from build123d import *

# Parameters (mm, degrees)
SKETCH_1_R      = 2
EXTRUDE_1_DEPTH = 3
FILLET_1_R      = 2
FILLET_2_R      = 5


with BuildPart() as part:
    # ｽｹｯﾁ1 → ﾎﾞｽ - 押し出し1 (new body)
    with BuildSketch(Plane(origin=(0, 0, 0), x_dir=(1, 0, 0), z_dir=(0, 1, 0))):
        Polygon((0, 20), (0, 160), (-10, 160), (-13.241161391, 160), (-45.078057301, 128.16310409), (-128.16310409, 45.078057301), (-160, 13.241161391), (-160, 10), (-160, 0), (-20, 0), align=None)
        with Locations(Location((-5, 25, 0), (0, 0, 270))):
            Circle(SKETCH_1_R, mode=Mode.SUBTRACT)
        with Locations(Location((-5, 90, 0), (0, 0, 270))):
            Circle(SKETCH_1_R, mode=Mode.SUBTRACT)
        with Locations(Location((-90, 5, 0), (0, 0, 270))):
            Circle(SKETCH_1_R, mode=Mode.SUBTRACT)
        with Locations(Location((-25, 5, 0), (0, 0, 270))):
            Circle(SKETCH_1_R, mode=Mode.SUBTRACT)
        with Locations(Location((-68.942911166, 97.227182413, 0), (0, 0, 270))):
            Circle(SKETCH_1_R, mode=Mode.SUBTRACT)
        with Locations(Location((-30.0520382, 58.336309448, 0), (0, 0, 270))):
            Circle(SKETCH_1_R, mode=Mode.SUBTRACT)
        with Locations(Location((-58.336309448, 30.0520382, 0), (0, 0, 270))):
            Circle(SKETCH_1_R, mode=Mode.SUBTRACT)
        with Locations(Location((-97.227182413, 68.942911166, 0), (0, 0, 270))):
            Circle(SKETCH_1_R, mode=Mode.SUBTRACT)
        with Locations(Location((-5, 155, 0), (0, 0, 270))):
            Circle(SKETCH_1_R, mode=Mode.SUBTRACT)
        with Locations(Location((-155, 5, 0), (0, 0, 270))):
            Circle(SKETCH_1_R, mode=Mode.SUBTRACT)
        Polygon((-82.201163313, 13.258252147), (-13.258252147, 82.201163313), (-45.078057301, 114.020968466), (-114.020968466, 45.078057301), align=None, mode=Mode.SUBTRACT)
    extrude(amount=EXTRUDE_1_DEPTH)

    # ﾌｨﾚｯﾄ1
    fillet_1_edges = [part.edges().sort_by_distance(p)[0] for p in [
        (-13.241161391, 1.5, -160),
        (0, 1.5, -160),
        (0, 1.5, -20),
        (-20, 1.5, 0),
        (-160, 1.5, 0),
        (-160, 1.5, -13.241161391),
    ]]
    fillet(fillet_1_edges, radius=FILLET_1_R)

    # ﾌｨﾚｯﾄ2
    fillet_2_edges = [part.edges().sort_by_distance(p)[0] for p in [
        (-82.201163313, 1.5, -13.258252147),
        (-13.258252147, 1.5, -82.201163313),
        (-45.078057301, 1.5, -114.020968466),
        (-114.020968466, 1.5, -45.078057301),
    ]]
    fillet(fillet_2_edges, radius=FILLET_2_R)


solid = part.part
Read the model definition and answer for the solid it produces. Units are mm, in the model's axes. A direction names the side the tool comes from. Give positions to 0.01 mm unless a question says otherwise; leave off trailing zeros. Write each loop counter-clockwise with the first axis right and the second up, starting at its lowest first coordinate (ties: lowest second). Pieces come first, ordered by that corner, then holes. Notation, with made-up numbers: M -6.75,59 L 16.25,59 A19 cw 16.25,74 Z; hole C 49.25,86 d3. An arc over 180 degrees is marked long. One line per item, written item: value. Start each with the question number.
(1) Find section A-A (z = -5). Determine the outline of the cut face in (x, y).
(2) A tool of negligible diameter and unlimited length cuts with its end or side. For faces 5 (the flat face through (-46, 0, -46)), 6 (the flat face through (-28.995, 1.479, -97.938)), from which of +Z, -Z, +X, -X, +Y, -Y can it reach the whole face along a straight path? Write none if from no direction.
(3) A flat-ended cylindrical pin translates along its axis: pin 1 Ø1 at (x, y) = (-17, 1.5) entering from +Z. Find the tip coordinate at first contact, or state that the pin passes through.
(4) Determine the mould class of faces 1 (the cylindrical face through (-59.102, 1.479, -28.205)), 2 (the flat face through (-46, 3, -46)), 3 (the flat face through (-85.6, 1.48, -87.64)), 4 (the flat face through (-10, 1, -10)) for opening direction Z: pulls with the +Z half, pulls with the -Z half, needs draft (parallel to the pull), parting line crosses it, or undercut.
(5) Find section B-B (x = -5). Determine the outline of the cut face in (y, z).
(6) Find section C-C (y = 2). Give the number of separate pieces and of enclosed holes in the cut face, plus the area to 3 significant figures.
(7) Find the intervals of material crossed by line 1 (X direction, y = 1.25, z = -5); line 2 (Z direction, x = -58.5, y = 2.7); line 3 (X direction, y = 1.05, z = -90), in increasing order.
(8) Find section D-D (z = -25). Determine the outline of the cut face in (x, y), plus the area to 3 significant figures.
Results below:
1. outline: M -160,0 L -157,0 L -157,3 L -160,3 Z; M -153,0 L -92,0 L -92,3 L -153,3 Z; M -88,0 L -27,0 L -27,3 L -88,3 Z; M -23,0 L -15,0 L -15,3 L -23,3 Z
2. face 5: +Z, -Z, +X, -X, -Y
2. face 6: +Y, -Y
3. pin 1: stops at z = -2.5
4. face 1: undercut
4. face 2: needs draft
4. face 3: pulls with the -Z half
4. face 4: pulls with the +Z half
5. outline: M 0,-160 L 3,-160 L 3,-157 L 0,-157 Z; M 0,-153 L 3,-153 L 3,-92 L 0,-92 Z; M 0,-88 L 3,-88 L 3,-27 L 0,-27 Z; M 0,-23 L 3,-23 L 3,-15 L 0,-15 Z
6. separate pieces: 1
6. enclosed holes: 11
6. area: 10,100 mm^2
7. line 1: x = -160 to -157, -153 to -92, -88 to -27, -23 to -15
7. line 2: z = -114.74 to -100.6, -36.96 to -32.05, -28.06 to 0
7. line 3: x = -83.24 to -69.1, -21.06 to -7, -3 to 0
8. outline: M -148.24,0 L -93.94,0 L -93.94,3 L -148.24,3 Z; M -70.46,0 L -7,0 L -7,3 L -70.46,3 Z; M -3,0 L 0,0 L 0,3 L -3,3 Z
8. area: 362 mm^2
